Solid Edge part; units mm, degrees
sketch "Sketch1" plane through (0, 0, 0) normal (0, -1, 0) x (1, 0, 0)
  arc A0 (11, 8.967) -> (13, 6.967) centre (11, 6.967) cw
  line L0 (13, 3.967) -> (13, 6.967)
  line L1 (13, 3.967) -> (14, 3)
  line L2 (14, 0) -> (14, 3)
  line L3 (0, 0) -> (14, 0)
  line L4 (0, 0) -> (0, 58.6569)
  line L5 (7, 42) -> (7, 44)
  arc A1 (5, 40) -> (7, 42) centre (5, 42) ccw
  arc A2 (11, 9.967) -> (9, 11.967) centre (9, 9.967) ccw
  line L6 (11, 8.967) -> (11, 9.967)
  arc A3 (0, 58.6569) -> (7, 44) centre (0, 49.6569) cw
  arc A4 (9, 11.967) -> (5, 40) centre (105, 39.9671) cw
revolve "RevolvedProtrusion1" add sketch "Sketch1" angle 360 about axis through (0, 0, 0) along (0, 0, 1)
The model under review builds one solid part; all positions refer to its coordinate system, in mm. A direction names the side the tool comes from. Coordinates: 2 decimals unless noted, no trailing zeros. Write each loop counter-clockwise with the first axis right and the second up, starting at its lowest first coordinate (ties: lowest second). Pieces come first, ordered by that corner, then holes. Notation, with made-up numbers: (17, 62) - (67, 62) arc R30 ccw to (67, 85) - close; hole circle Ø2 at (56.25, 1.25). An arc over 180 degrees is marked (long way). Answer as a JSON object with one key per item and string values. Group by question number.
1. Mouldability with a two-part tool opening along Z and no side actions: class faces 1 (the face through (0, 0, 0)), 2 (the face through (-2.38, -10.74, 9.47)), 3 (the face through (6.466, -2.681, 43.014)) as pulls with the +Z half, pulls with the -Z half, needs draft (parallel to the pull), parting line crosses it, or undercut.
2. Add section B-B (z = 6). Give the boundary of the cut face in (x, y), plus the area to 3 significant figures.
3. Add section A-A (y = 0). Give the boundary of the cut face in (x, z).
4. Add section D-D (z = 23). Give the boundary of the cut face in (x, y).
5. To check wall thickness, follow probe 1 along Z at (x, y) = (-7.25, -5.5); probe 2 along X at (y, z) = (-6.5, 8.5); probe 3 along X at (y, z) = (-2, 20.5). State the ranges of each line that lie inside material, in increasing order.
6. Clearance check with flat-ended pins moving along their axes: pin 1 Ø5 at (y, z) = (-3.5, 24.5) entering from -X; pin 2 Ø3 at (x, y) = (-10, -11) entering from +Z; pin 3 Ø1 at (y, z) = (5.5, 31) entering from +X. State where each tip first meets the part, or that it passes through.
7. Machinability: for faces 4 (the face through (12.932, -5.362, 1.521)), 5 (the face through (-10.316, -7.91, 5.488)), which of the approach directions +Z, -Z, +X, -X, +Y, -Y give a long, thin tool a straight path to every point of the face, cutting with its end or side? Answer none if there is none.
Findings:
{
 "1": {"face 1": "pulls with the -Z half", "face 2": "needs draft", "face 3": "undercut"},
 "2": {"outline": "circle Ø26 at (0, 0)", "area": "531 mm²"},
 "3": {"outline": "(-14, 0) - (14, 0) - (14, 3) - (13, 3.97) - (13, 6.97) arc R2 ccw to (11, 8.97) - (11, 9.97) arc R2 ccw to (9, 11.97) arc R100 cw to (5, 40) arc R2 ccw to (7, 42) - (7, 44) arc R9 ccw (long way) to (-7, 44) - (-7, 42) arc R2 ccw to (-5, 40) arc R100 cw to (-9, 11.97) arc R2 ccw to (-11, 9.97) - (-11, 8.97) arc R2 ccw to (-13, 6.97) - (-13, 3.97) - (-14, 3) - close"},
 "4": {"outline": "circle Ø12.9 at (0, 0)"},
 "5": {"probe 1": "0 to 11.96", "probe 2": "-10.42 to 10.42", "probe 3": "-6.62 to 6.62"},
 "6": {"pin 1": "x = -6.27", "pin 2": "z = 3.61", "pin 3": "x = 2.05"},
 "7": {"face 4": "+Z, -Z", "face 5": "+Z"}
}
